Study the drawing (mm; zero at the part's minimum x, y, z) and answer. Coordinates: 2 decimals unless noted, no trailing zeros. Order: outer loops, then holes, each group sorted by start corner. A loop starts at its lowest first (then second) coordinate and runs counter-clockwise, first axis right, second up.
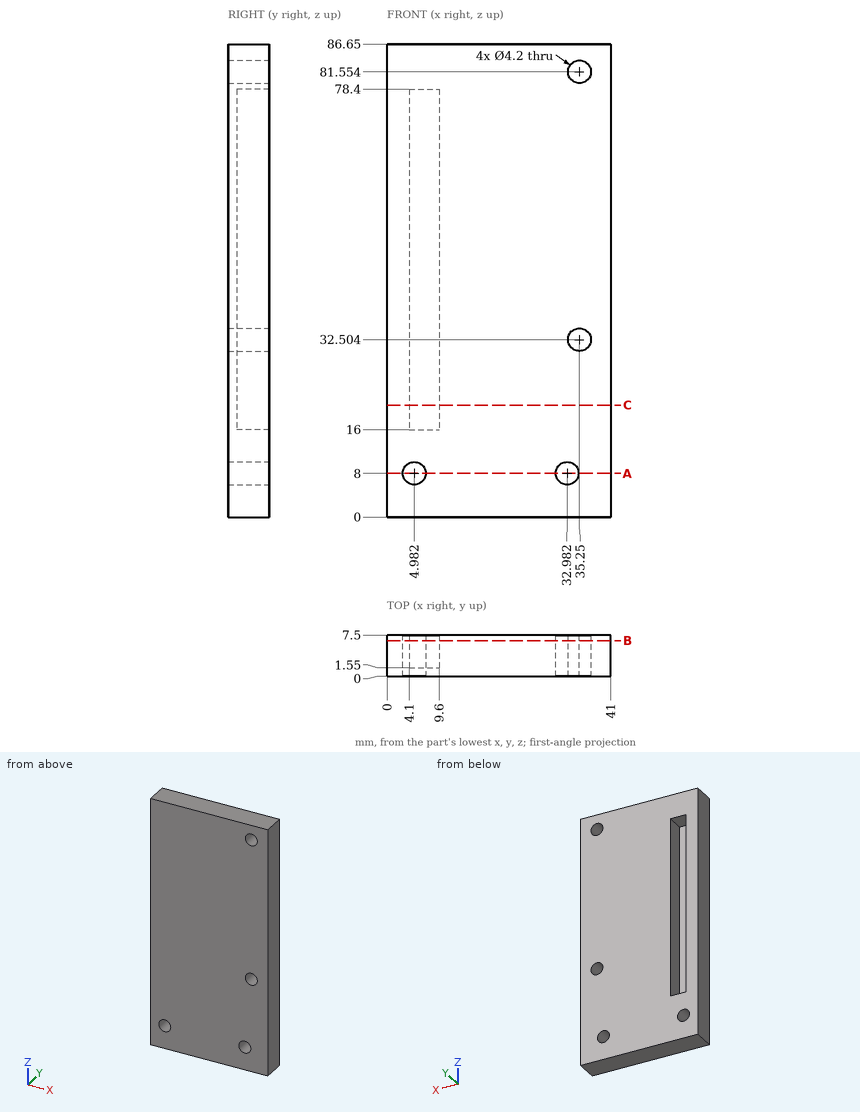
(1) Find section C-C on z = 20.5. Determine the outline of the cut face in (x, y), then the cut area to 3 significant figures.
(2) Find section A-A on z = 8. Determine the outline of the cut face in (x, y).
(3) Find section B-B on y = 6.5. Determine the outline of the cut face in (x, z), then the cut area to 3 significant figures.
(4) Given pin 1 Ø6.5 at (x, z) = (35.25, 81.554) entering from -Y; pin 2 Ø3 at (x, z) = (6, 51) entering from +Y, each flat-ended and moving along its own axis, determine where each tip first touches the part or whether it passes through.
(5) Find the intervals of material crossed by probe 1 along Z at (x, y) = (35.25, 4.75); probe 2 along X at (y, z) = (3.25, 8); probe 3 along X at (y, z) = (2.5, 43), in increasing order.
Resolved:
1. outline: (0, 0) - (41, 0) - (41, 7.5) - (9.6, 7.5) - (9.6, 1.55) - (4.1, 1.55) - (4.1, 7.5) - (0, 7.5) - close
1. area: 275 mm2
2. outline: (0, 0) - (2.88, 0) - (2.88, 7.5) - (0, 7.5) - close; (7.08, 0) - (30.88, 0) - (30.88, 7.5) - (7.08, 7.5) - close; (35.08, 0) - (41, 0) - (41, 7.5) - (35.08, 7.5) - close
3. outline: (0, 0) - (41, 0) - (41, 86.65) - (0, 86.65) - close; hole circle Ø4.2 at (4.98, 8); hole (4.1, 16) - (9.6, 16) - (9.6, 78.4) - (4.1, 78.4) - close; hole circle Ø4.2 at (32.98, 8); hole circle Ø4.2 at (35.25, 32.5); hole circle Ø4.2 at (35.25, 81.55)
3. area: 3,150 mm2
4. pin 1: stops at y = 0
4. pin 2: stops at y = 1.55
5. probe 1: z = 0 to 30.4, 34.6 to 79.45, 83.65 to 86.65
5. probe 2: x = 0 to 2.88, 7.08 to 30.88, 35.08 to 41
5. probe 3: x = 0 to 4.1, 9.6 to 41
